```python
from build123d import *

# Parameters (mm, degrees)
BOSS_EXTRUDE1_DEPTH         = 5
SHELL1_T                    = -0.5
SKETCH4_R                   = 2.5
CUT_EXTRUDE4_DEPTH          = 10
CUT_SWEEP2_START            = 1
CUT_SWEEP2_DEPTH            = 4
SKETCH8_W                   = 6
SKETCH8_H                   = 10.878336181
CUT_EXTRUDE6_DEPTH          = 10
SKETCH11_R                  = 4.5
SKETCH11_R_2                = 10.5
SKETCH11_R_3                = 10
CUT_EXTRUDE7_DEPTH          = 150.877510373
FILLET1_R                   = 1
BOSS_EXTRUDE6_START         = 69.993050043
BOSS_EXTRUDE6_DEPTH         = 26.446393474
BOSS_EXTRUDE6_START_2       = -40
BOSS_EXTRUDE6_2_OUTLINE_W   = 1.69894254
BOSS_EXTRUDE6_2_OUTLINE_H   = 3
BOSS_EXTRUDE6_2_OUTLINE_W_2 = 1.590498846
BOSS_EXTRUDE6_2_OUTLINE_H_2 = 10
BOSS_EXTRUDE6_2_DEPTH       = 7.043773978
BOSS_EXTRUDE6_3_OUTLINE_W   = 1.69894254
BOSS_EXTRUDE6_3_OUTLINE_H   = 7
BOSS_EXTRUDE6_3_DEPTH       = 3.122658049
BOSS_EXTRUDE6_START_3       = -33.015543653
BOSS_EXTRUDE6_4_OUTLINE_W   = 1.590498846
BOSS_EXTRUDE6_4_OUTLINE_H   = 3
BOSS_EXTRUDE6_4_DEPTH       = 2.015543653
SKETCH17_R                  = 3
CUT_EXTRUDE8_DEPTH          = 10
CUT_EXTRUDE9_DEPTH          = 10
SKETCH19_R                  = 2
CUT_EXTRUDE10_DEPTH         = 150.877510373
CUT_EXTRUDE11_DEPTH         = 10


with BuildPart() as part:
    # Sketch1 → Boss-Extrude1 (new, symmetric)
    with BuildSketch(Plane.XY):
        with BuildLine():
            Line((0, 0), (64, 0))
            Line((64, 0), (57.458864255, 46.542599231))
            ThreePointArc((57.458864255, 46.542599231), (60.521124606, 56.88061692), (70.332349149, 61.351849543))
            Line((70.332349149, 61.351849543), (81.602015886, 61.351849543))
            ThreePointArc((81.602015886, 61.351849543), (85.0970904, 61.9825137), (88.15132127, 63.794958715))
            Line((88.15132127, 63.794958715), (95.587384775, 70.239547086))
            ThreePointArc((95.587384775, 70.239547086), (98.399557697, 74.280371374), (98.942828678, 79.173369852))
            Line((98.942828678, 79.173369852), (96.783267224, 94.707844854))
            ThreePointArc((96.783267224, 94.707844854), (95.173069343, 98.916646259), (91.878517937, 101.991166954))
            Line((91.878517937, 101.991166954), (76.780291664, 110.708131957))
            ThreePointArc((76.780291664, 110.708131957), (74.368482115, 111.707136182), (71.780291664, 112.047877919))
            Line((71.780291664, 112.047877919), (15.23328628, 112.047877919))
            ThreePointArc((15.23328628, 112.047877919), (10.23328628, 110.708131957), (6.573032242, 107.047877919))
            Line((6.573032242, 107.047877919), (-5.979384502, 85.30645436))
            ThreePointArc((-5.979384502, 85.30645436), (-7.273805779, 79.355434178), (-4.876021292, 73.757148976))
            Line((-4.876021292, 73.757148976), (2.24853328, 65.536509085))
            ThreePointArc((2.24853328, 65.536509085), (6.355355668, 62.120008219), (8.572429973, 57.259653311))
            Line((8.572429973, 57.259653311), (0, 8))
            Line((0, 8), (0, 0))
        make_face()
    extrude(amount=BOSS_EXTRUDE1_DEPTH, both=True)

    # Shell1
    shell1_openings = [part.faces().sort_by_distance(p)[0] for p in [
        (40.493150865, 62.038987827, 5),
    ]]
    offset(amount=SHELL1_T, openings=shell1_openings, kind=Kind.INTERSECTION)

    # Sketch4 → Cut-Extrude4 (cut)
    with BuildSketch(Plane.XZ):
        with Locations(Location((7, 0, 0), (0, 0, 270))):
            Circle(SKETCH4_R)
        with Locations(Location((57, 0, 0), (0, 0, 270))):
            Circle(SKETCH4_R)
        with BuildLine():
            Line((23, 5), (35, 5))
            ThreePointArc((35, 5), (29, 3.5), (23, 5))
        make_face()
    extrude(amount=-CUT_EXTRUDE4_DEPTH, mode=Mode.SUBTRACT)

    # Cut-Sweep2: read off the stored shape, not the designer's step
    # Cut-Sweep2 outline → Cut-Sweep2 (cut)
    with BuildSketch(Plane.XY.offset(CUT_SWEEP2_START)):
        with BuildLine():
            Line((63.222895016, 0.5), (63.293165433, 0))
            Line((63.293165433, 0), (64, 0))
            Line((64, 0), (57.458864255, 46.542599231))
            ThreePointArc((57.458864255, 46.542599231), (60.521124606, 56.88061692), (70.332349149, 61.351849543))
            Line((70.332349149, 61.351849543), (81.602015886, 61.351849543))
            ThreePointArc((81.602015886, 61.351849543), (85.0970904, 61.9825137), (88.15132127, 63.794958715))
            Line((88.15132127, 63.794958715), (95.587384775, 70.239547086))
            ThreePointArc((95.587384775, 70.239547086), (98.399557697, 74.280371374), (98.942828678, 79.173369852))
            Line((98.942828678, 79.173369852), (96.783267224, 94.707844854))
            ThreePointArc((96.783267224, 94.707844854), (95.173069343, 98.916646258), (91.878517937, 101.991166954))
            Line((91.878517937, 101.991166954), (76.780291664, 110.708131957))
            ThreePointArc((76.780291664, 110.708131957), (74.368482115, 111.707136182), (71.780291664, 112.047877919))
            Line((71.780291664, 112.047877919), (15.23328628, 112.047877919))
            ThreePointArc((15.23328628, 112.047877919), (10.23328628, 110.708131957), (6.573032242, 107.047877919))
            Line((6.573032242, 107.047877919), (-5.979384502, 85.30645436))
            ThreePointArc((-5.979384502, 85.30645436), (-7.273805779, 79.355434178), (-4.876021292, 73.757148976))
            Line((-4.876021292, 73.757148976), (2.24853328, 65.536509085))
            ThreePointArc((2.24853328, 65.536509085), (6.355355668, 62.120008219), (8.572429973, 57.259653311))
            Line((8.572429973, 57.259653311), (0, 8))
            Line((0, 8), (0, 0.5))
            Line((0, 0.5), (0.5, 0.5))
            Line((0.5, 0.5), (0.5, 7.956818155))
            Line((0.5, 7.956818155), (9.081153751, 57.266600812))
            ThreePointArc((9.081153751, 57.266600812), (6.811556982, 62.345857113), (2.562843108, 65.937283639))
            Line((2.562843108, 65.937283639), (-4.498176751, 74.084614245))
            ThreePointArc((-4.498176751, 74.084614245), (-6.776072013, 79.402985187), (-5.5463718, 85.05645436))
            Line((-5.5463718, 85.05645436), (7.006044944, 106.797877919))
            ThreePointArc((7.006044944, 106.797877919), (10.48328628, 110.275119255), (15.23328628, 111.547877919))
            Line((15.23328628, 111.547877919), (71.780291664, 111.547877919))
            ThreePointArc((71.780291664, 111.547877919), (74.239072592, 111.224173269), (76.530291664, 110.275119255))
            Line((76.530291664, 110.275119255), (91.628517937, 101.558154252))
            ThreePointArc((91.628517937, 101.558154252), (94.758341773, 98.637359591), (96.28802976, 94.638998257))
            Line((96.28802976, 94.638998257), (98.447591213, 79.104523255))
            ThreePointArc((98.447591213, 79.104523255), (97.931483782, 74.456174701), (95.259919506, 70.617391628))
            Line((95.259919506, 70.617391628), (87.823856001, 64.172803257))
            ThreePointArc((87.823856001, 64.172803257), (84.922336675, 62.450980492), (81.602015886, 61.851849543))
            Line((81.602015886, 61.851849543), (70.332349149, 61.851849543))
            ThreePointArc((70.332349149, 61.851849543), (60.143769816, 57.208646435), (56.963730221, 46.47301268))
            Line((56.963730221, 46.47301268), (63.424815796, 0.5))
            Line((63.424815796, 0.5), (63.222895016, 0.5))
        make_face()
    extrude(amount=CUT_SWEEP2_DEPTH, mode=Mode.SUBTRACT)

    # Sketch8 → Cut-Extrude6 (cut)
    with BuildSketch(Plane(origin=(34.097487332, 29.551155688, 0), x_dir=(0, 0, -1), z_dir=(0.7556890827898172, 0.6549305384178423, 0))):
        with Locations((2, 53.491759419)):
            Rectangle(SKETCH8_W, SKETCH8_H)
    extrude(amount=-CUT_EXTRUDE6_DEPTH, mode=Mode.SUBTRACT)

    # Sketch11 → Cut-Extrude7 (cut, through all)
    with BuildSketch(Plane.XY.offset(5)):
        with Locations(Location((21.843413851, 65.071690598, 0), (0, 0, 180))):
            Circle(SKETCH11_R)
        with Locations(Location((60.516838143, 83.547877919, 0), (0, 0, 180))):
            Circle(SKETCH11_R_2)
        with Locations(Location((35.016838143, 83.547877919, 0), (0, 0, 180))):
            Circle(SKETCH11_R_3)
    extrude(amount=-CUT_EXTRUDE7_DEPTH, mode=Mode.SUBTRACT)

    # Fillet1
    # the kernel refuses this fillet: 1 mm, written as the material it takes off along each edge
    with BuildSketch(Plane(origin=(60.516838143, 83.547877919, -4.5), x_dir=(-1, 0, 0), z_dir=(0, 1, 0))) as fillet1_piece_1:
        with BuildLine():
            CenterArc((11.366025404, -1), FILLET1_R, 90, 60)
            Line((11.366025404, 0), (11.366025404, 0.02))
            Line((11.366025404, 0.02), (10.5, 0.02))
            Line((10.5, 0.02), (10.48, 0))
            ThreePointArc((10.48, 0), (10.48, -0.25), (10.482679492, -0.49))
            Line((10.482679492, -0.49), (10.5, -0.5))
        make_face()
    revolve(axis=Axis((60.516838143, 83.547877919, -4.5), (0, 0, 1)), mode=Mode.SUBTRACT)

    # Boss-Extrude6: read off the stored shape, not the designer's step
    # Boss-Extrude6 outline → Boss-Extrude6 (add)
    with BuildSketch(Plane(origin=(0, 0, 0), x_dir=(0.8660254037844399, -0.4999999999999979, 0), z_dir=(0.4999999999999979, 0.8660254037844398, 0)).offset(BOSS_EXTRUDE6_START)):
        with BuildLine():
            add(Edge.make_bspline(
                [(-47.337092239, -1), (-47.337092239, -2.5), (-48.820393697, -2.5), (-50.303695156, -2.5), (-50.303695156, -1)],
                knots=[0, 0, 0, 1.570796327, 1.570796327, 3.141592654, 3.141592654, 3.141592654], degree=2, weights=[1, 0.707106781, 1, 0.707106781, 1]))
            Line((-47.337092239, -1), (-47.831526058, -1))
            add(Edge.make_bspline(
                [(-47.831526058, -1), (-47.831526058, -2), (-48.820393697, -2), (-49.809261336, -2), (-49.809261336, -1)],
                knots=[0, 0, 0, 1.570796327, 1.570796327, 3.141592654, 3.141592654, 3.141592654], degree=2, weights=[1, 0.707106781, 1, 0.707106781, 1]))
            Line((-49.809261336, -1), (-49.809261336, 4))
            Line((-49.809261336, 4), (-50.303695156, 4))
            Line((-50.303695156, 4), (-50.303695156, -1))
        make_face()
    extrude(amount=BOSS_EXTRUDE6_DEPTH)

    # Boss-Extrude6 2 outline → Boss-Extrude6 2 (cut)
    with BuildSketch(Plane(origin=(0, 0, 0), x_dir=(0.365571123575949, 0.9307834085368187, 0), z_dir=(0.9307834085368187, -0.36557112357594895, 0)).offset(BOSS_EXTRUDE6_START_2)):
        with Locations((75.84947127, 2.5)):
            Rectangle(BOSS_EXTRUDE6_2_OUTLINE_W, BOSS_EXTRUDE6_2_OUTLINE_H)
        with Locations((103.204750577, -1)):
            Rectangle(BOSS_EXTRUDE6_2_OUTLINE_W_2, BOSS_EXTRUDE6_2_OUTLINE_H_2)
    extrude(amount=BOSS_EXTRUDE6_2_DEPTH, mode=Mode.SUBTRACT)

    # Boss-Extrude6 3 outline → Boss-Extrude6 3 (cut)
    with BuildSketch(Plane(origin=(0, 0, 0), x_dir=(0.365571123575949, 0.9307834085368187, 0), z_dir=(0.9307834085368187, -0.36557112357594895, 0)).offset(BOSS_EXTRUDE6_START_2)):
        with Locations((75.84947127, -2.5)):
            Rectangle(BOSS_EXTRUDE6_3_OUTLINE_W, BOSS_EXTRUDE6_3_OUTLINE_H)
    extrude(amount=BOSS_EXTRUDE6_3_DEPTH, mode=Mode.SUBTRACT)

    # Boss-Extrude6 4 outline → Boss-Extrude6 4 (cut)
    with BuildSketch(Plane(origin=(0, 0, 0), x_dir=(0.365571123575949, 0.9307834085368187, 0), z_dir=(0.9307834085368187, -0.36557112357594895, 0)).offset(BOSS_EXTRUDE6_START_3)):
        with Locations((103.204750577, 2.5)):
            Rectangle(BOSS_EXTRUDE6_4_OUTLINE_W, BOSS_EXTRUDE6_4_OUTLINE_H)
    extrude(amount=BOSS_EXTRUDE6_4_DEPTH, mode=Mode.SUBTRACT)

    # Sketch17 → Cut-Extrude8 (cut)
    with BuildSketch(Plane(origin=(0, 0, -5), x_dir=(-1, 0, 0), z_dir=(0, 0, -1))):
        with Locations((-86.847845229, 80.771032583)):
            Circle(SKETCH17_R)
        with Locations((-15.370383265, 103.018842591)):
            Circle(SKETCH17_R)
    extrude(amount=-CUT_EXTRUDE8_DEPTH, mode=Mode.SUBTRACT)

    # Sketch18 → Cut-Extrude9 (cut)
    with BuildSketch(Plane.XY.offset(-4.5)):
        Polygon((67.794990984, 63.159599672), (67.758803504, 62.660910926), (73.743068466, 62.226661163), (73.779255946, 62.72534991), align=None)
        Polygon((76.601879403, 101.623072167), (76.638066884, 102.121760914), (70.653801921, 102.556010677), (70.617614441, 102.05732193), align=None)
        Polygon((22.614883225, 103.298241446), (22.364883225, 102.865228744), (29.293086455, 98.865228744), (29.543086455, 99.298241446), align=None)
        Polygon((14.659111859, 71.518441227), (7.730908628, 75.518441227), (7.480908628, 75.085428525), (14.409111859, 71.085428525), align=None)
    extrude(amount=-CUT_EXTRUDE9_DEPTH, mode=Mode.SUBTRACT)

    # Sketch19 → Cut-Extrude10 (cut, through all)
    with BuildSketch(Plane(origin=(0, 0, -5), x_dir=(-1, 0, 0), z_dir=(0, 0, -1))):
        with Locations((-57.950079932, 60)):
            Circle(SKETCH19_R)
        with Locations((-35.950079932, 60)):
            Circle(SKETCH19_R)
    extrude(amount=-CUT_EXTRUDE10_DEPTH, mode=Mode.SUBTRACT)

    # Sketch20 → Cut-Extrude11 (cut)
    with BuildSketch(Plane(origin=(0, 0, -5), x_dir=(-1, 0, 0), z_dir=(0, 0, -1))):
        Polygon((-91.592738232, 89.181501678), (-91.308182839, 87.201848115), (-84.379395369, 88.19779199), (-84.663950762, 90.177445553), align=None)
        Polygon((-89.316295089, 73.344273176), (-89.031739697, 71.364619614), (-82.102952227, 72.360563488), (-82.38750762, 74.340217051), align=None)
    extrude(amount=-CUT_EXTRUDE11_DEPTH, mode=Mode.SUBTRACT)


solid = part.part
```
For this review, take the finished solid that the model builds, in its own axes (mm). A direction names the side the tool comes from. Round coordinates to 2 decimals unless told otherwise and drop trailing zeros. Write each loop counter-clockwise with the first axis right and the second up, starting at its lowest first coordinate (ties: lowest second). Pieces come first, ordered by that corner, then holes. Notation, with made-up numbers: (-15.5, 60.25) -> (22.5, 60.25) arc R15 cw to (22.5, 80.25) -> close; hole circle Ø11 at (-11.75, -9). An arc over 180 degrees is marked (long way). Use one line per item in the form item = value.
Q1. Consider section C-C (y = 13). State the section outline as (x, z) points.
Resolved:
outline = (0.87, -5) -> (62.17, -5) -> (62.17, 1) -> (61.67, 1) -> (61.67, -4.5) -> (1.38, -4.5) -> (1.38, 1) -> (0.87, 1) -> close
Q2. Machinability: for faces 4 (the cylindrical face through (74.273, 111.215, -1.712)), 5 (the flat face through (-1.69, 96.69, -1.47)), 6 (the flat face through (-1.9, 96.8, -4)), 7 (the cylindrical face through (4.78, 0.25, -1.15)), which of the approach directions +Z, -Z, +X, -X, +Y, -Y give a long, thin tool a straight path to every point of the face, cutting with its end or side? Answer none if there is none.
Resolved:
face_4 = +Z
face_5 = -Z
face_6 = -Z, -X, +Y
face_7 = -Y
Q3. Consider section B-B (x = 39.5). State the section outline as (y, z) points.
Resolved:
outline = (0, -5) -> (74.61, -5) -> (74.61, -4.5) -> (0.5, -4.5) -> (0.5, 5) -> (0, 5) -> close; (92.49, -5) -> (112.05, -5) -> (112.05, 1) -> (111.55, 1) -> (111.55, -4.5) -> (92.49, -4.5) -> close
Q4. The part is to be moulded in two halves that separate along Z. For faces 1 (the cylindrical face through (97.908, 74.394, -1.712)), 2 (the flat face through (5.19, 35.79, 1)), 3 (the cylindrical face through (54.56, 0.25, 0.54)), say which applies: released by +Z, released by -Z, zero draft, split by the parting line, or undercut.
Resolved:
face_1 = zero draft
face_2 = released by +Z
face_3 = undercut
Q5. Consider section D-D (y = 30). State the section outline as (x, z) points, then the cut area to 3 significant figures.
Resolved:
outline = (3.83, -5) -> (59.78, -5) -> (59.78, 1) -> (59.28, 1) -> (59.28, -4.5) -> (4.34, -4.5) -> (4.34, 1) -> (3.83, 1) -> close
area = 33.5 mm²
Q6. To check wall thickness, follow probe 1 along Y at (x, z) = (47, 0); probe 2 along X at (y, z) = (0.3, 0); probe 3 along X at (y, z) = (102, -2.5). State the ranges of each line that lie inside material, in increasing order. Write a range as from..to.
Resolved:
probe_1 = 0..0.5, 111.55..112.05
probe_2 = 0..4.5, 9.5..54.5, 59.5..63.96
probe_3 = 0.8..1.37, 3.66..4.24, 90.86..91.86
Q7. Clearance check with flat-ended pins moving along their axes: pin 1 Ø6 at (y, z) = (43.5, -2.5) entering from +X; pin 2 Ø10 at (x, y) = (4, 30) entering from +Z; pin 3 Ø2 at (x, y) = (46, 33.5) entering from +Z; pin 4 Ø5.5 at (x, y) = (86.85, 80.77) entering from +Z. State where each tip first meets the part, or that it passes through.
Resolved:
pin_1 = 58.31
pin_2 = 1
pin_3 = -4.5
pin_4 = through
Q8. Consider section A-A (y = 67.5). State the section outline as (x, z) points.
Resolved:
outline = (1.21, -5) -> (18.05, -5) -> (18.05, -4.5) -> (1.21, -4.5) -> close; (25.63, -5) -> (92.43, -5) -> (92.43, 1) -> (91.66, 1) -> (91.66, -4.5) -> (25.63, -4.5) -> close
